Input: part model. Units: mm. Frame: model coordinates. Face numbers are marked on the shaded views. A direction names the side the tool comes from. Coordinates: 2 decimals unless noted, no trailing zeros. Write each loop counter-clockwise with the first axis right and the second up, starting at its lowest first coordinate (ties: lowest second). Pieces come first, ordered by that corner, then holes. Notation, with made-up numbers: M 41,76 L 98,76 A32 ccw 98,105 Z; hole C -10.5,31 d7. An arc over 180 degrees is marked long. Write each question's results on one line, items separated by ' | '. Start each with the question number.
1. First-contact query: pin 1 (2 mm diameter, centred on y = -2, z = 13, fed in from +X); pin 2 (4 mm diameter, centred on y = -4, z = 25, fed in from +X); pin 3 (4 mm diameter, centred on x = 0.5, z = 28.5, fed in from +Y). Flat tips, straight axial feed; report the tip coordinate or a pass-through.
2. Section query D-D, the plane z = 11.5. Output: boundary loops of the cut face in (x, y), and give its area (3 significant figures).
3. Section query A-A, the plane x = 0. Output: boundary loops of the cut face in (y, z).
4. Ray query, probe 1 along Z at (x, y) = (1.5, 4.25); probe 2 along Y at (x, z) = (0.25, 6); probe 3 along Y at (x, z) = (1.75, 18). Return the intervals inside material, ascending.
5. Section query C-C, the plane z = 31.5. Output: boundary loops of the cut face in (x, y), and give its area (3 significant figures).
6. Set-up query: the marked faces 1, 2 and 3. Return all of +Z, -Z, +X, -X, +Y, -Y with unobstructed straight access to the full face (end or side cutting, diameter ignored); none if empty.
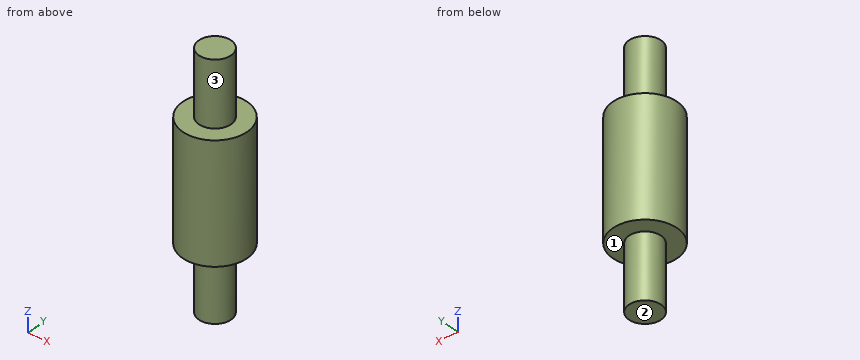
Autodesk Fusion 360 part; units mm, degrees
sketch "Esquisse1" plane through (0, 0, 0) normal (0, 0, 1) x (1, 0, 0)
  circle A0 centre (0, 0) radius 6
  dimension "d1" = 12
extrude "Extrusion1" add sketch "Esquisse1" along normal blind 22
sketch "Esquisse2" plane through (0, 0, 22) normal (0, 0, 1) x (-1, 0, 0)
  circle A0 centre (0, 0) radius 6
  circle A1 centre (0, 0) radius 3
  dimension "d4" = 6
extrude "Extrusion2" add sketch "Esquisse2" along normal blind 12 contours A1
sketch "Esquisse3" plane through (0, 0, 0) normal (0, 0, -1) x (1, 0, 0)
  circle A0 centre (0, 0) radius 6
  circle A1 centre (0, 0) radius 3
  dimension "d7" = 6
extrude "Extrusion3" add sketch "Esquisse3" along normal blind 12 contours A1
Answer:
1) pin 1: x = 5.92 | pin 2: x = 2.24 | pin 3: y = 3
2) outline: C 0,0 d12 | area: 113 mm^2
3) outline: M -6,0 L -3,0 L -3,-12 L 3,-12 L 3,0 L 6,0 L 6,22 L 3,22 L 3,34 L -3,34 L -3,22 L -6,22 Z
4) probe 1: 0 to 22 | probe 2: -5.99 to 5.99 | probe 3: -5.74 to 5.74
5) outline: C 0,0 d6 | area: 28.3 mm^2
6) face 1: -Z | face 2: -Z, +X, -X, +Y, -Y | face 3: +Z
